Autodesk Inventor part; units mm, degrees
ref_plane "YZ Plane" through (0, 0, 0) normal (1, 0, 0) x (0, 1, 0)
ref_plane "XZ Plane" through (0, 0, 0) normal (0, 1, 0) x (-1, 0, 0)
ref_plane "XY Plane" through (0, 0, 0) normal (0, 0, 1) x (1, 0, 0)
sketch "Skizze_Grudnkörper" plane through (0, 0, 0) normal (0, 0, 1) x (1, 0, 0)
  line L0 (-56, 0) -> (56, 0)
  line L1 (0, -12.6) -> (0, 12.6)
  line L2 (40, -9) -> (-40, -9)
  line L3 (-40, -9) -> (-40, 9)
  line L4 (-40, 9) -> (40, 9)
  line L5 (40, 9) -> (40, -9)
  line L6 (40, -9) -> (-40, 9) construction
  line L7 (-40, -9) -> (40, 9) construction
  point P0 (0, 0)
  dimension "Länge" = 80
  dimension "Breite" = 18
extrude "Grundkörper" add sketch "Skizze_Grudnkörper" along normal blind 10
sketch "Skizze_Senkbohrung" plane through (0, 0, 10) normal (0, 0, 1) x (1, 0, 0)
  line L0 (-56, 0) -> (56, 0)
  line L1 (0, -12.6) -> (0, 12.6)
  line L2 (-40, -9) -> (40, -9)
  line L3 (40, -9) -> (40, 9)
  line L4 (40, 9) -> (-40, 9)
  line L5 (-40, 9) -> (-40, -9)
  point P0 (0, 0)
  point P1 (-35, 0)
  point P2 (35, 0)
  dimension "d4" = 70
hole "Senkbohrung" at (-35, 0, 10) at (35, 0, 10) direction (0, 0, -1) diameter 4.5 end through all counterbore diameter 8 counterbore depth 4.6
sketch "Skizze_Ausnehmung" plane through (0, 0, 0) normal (0, 0, -1) x (-1, 0, 0)
  circle A0 centre (35, 0) radius 2.25
  circle A1 centre (-35, 0) radius 2.25
  line L0 (-40, -9) -> (40, -9)
  line L1 (40, -9) -> (40, 9)
  line L2 (40, 9) -> (-40, 9)
  line L3 (-40, 9) -> (-40, -9)
  line L4 (56, 0) -> (-56, 0)
  line L5 (0, -12.6) -> (0, 12.6)
  line L6 (40, 9) -> (-40, 9)
  line L7 (40, -9) -> (30, -9)
  line L8 (30, -9) -> (30, 9)
  line L9 (30, 9) -> (40, 9)
  line L10 (40, 9) -> (40, -9)
  line L11 (-40, 9) -> (-40, -9)
  line L12 (-40, -9) -> (-30, -9)
  line L13 (-30, -9) -> (-30, 9)
  line L14 (-30, 9) -> (-40, 9)
  line L15 (-40, 9) -> (-40, -9)
  point P0 (0, 0)
  dimension "d12" = 60
extrude "Ausnehmung" cut sketch "Skizze_Ausnehmung" against normal blind 2 contours L4 L1 L0 L8 A0 | A0 L4 L8 L2 L1 | L13 L0 L3 L4 A1 | L4 A1 L3 L2 L13
properties material "Stahl, unlegiert"
Check sheet for the modelled part. Datum: model origin and axes. Units: mm. A direction names the side the tool comes from. Coordinates: 2 decimals unless noted, no trailing zeros. Loops run counter-clockwise (first coordinate to the right, second up) from the corner with the lowest first, then second, coordinate; pieces in that order, holes last.
1) Gauge pin test, flat ends, axial feed: pin 1 (10.5 mm diameter, centred on x = 35, y = 0, fed in from +Z); pin 2 (1.6 mm diameter, centred on y = -0.5, z = 0.5, fed in from -X); pin 3 (7 mm diameter, centred on x = -35, y = 0, fed in from +Z); pin 4 (3 mm diameter, centred on x = -37.5, y = 3.5, fed in from -Z). Record the tip position at first contact, or that the pin passes through.
2) Sectioned sample at C-C (z = 6.75). Record the boundary of the cut face in (x, y).
3) Access from +Z, -Z, +X, -X, +Y, -Y to the whole of each face (thin tool, end or side, straight path). Record for faces 4 (the face through (-33.8, 2.1, 2)), 5 (the face through (37, -2, 5.4)), 6 (the face through (-37.23, 0.29, 3.68)), 7 (the face through (36.2, 2.1, 2)), 8 (the face through (-40, 0, 6)).
4) Release check for a two-part mould opening along Y. For faces 1 (the face through (-30, 0, 1)), 2 (the face through (1, -9, 5)), 3 (the face through (32.77, 0.29, 3.68)) record: released by +Y, released by -Y, zero draft, split by the parting line, or undercut.
5) Sectioned sample at B-B (x = -35). Record the boundary of the cut face in (y, z), and give its area (3 significant figures).
6) Material ranges on probe 1 along X at (y, z) = (0, 6.85); probe 2 along Y at (x, z) = (-35, 2.8); probe 3 along Y at (x, z) = (-35, 8.15), recorded low to high.
7) Sectioned sample at A-A (y = 0). Record the boundary of the cut face in (x, z), and give its area (3 significant figures).
8) Sectioned sample at D-D (z = 1). Record the boundary of the cut face in (x, y).
Check sheet entries:
1. pin 1: stops at z = 10
1. pin 2: stops at x = -30
1. pin 3: stops at z = 5.4
1. pin 4: stops at z = 2
2. outline: (-40, -9) - (40, -9) - (40, 9) - (-40, 9) - close; hole circle Ø8 at (-35, 0); hole circle Ø8 at (35, 0)
3. face 4: -Z, -X, +Y, -Y
3. face 5: +Z
3. face 6: +Z, -Z
3. face 7: -Z, +X, +Y, -Y
3. face 8: +Z, -Z, -X, +Y, -Y
4. face 1: zero draft
4. face 2: released by -Y
4. face 3: undercut
5. outline: (-9, 2) - (-2.25, 2) - (-2.25, 5.4) - (-4, 5.4) - (-4, 10) - (-9, 10) - close; (2.25, 2) - (9, 2) - (9, 10) - (4, 10) - (4, 5.4) - (2.25, 5.4) - close
5. area: 91.9 mm2
6. probe 1: x = -40 to -39, -31 to 31, 39 to 40
6. probe 2: y = -9 to -2.25, 2.25 to 9
6. probe 3: y = -9 to -4, 4 to 9
7. outline: (-40, 2) - (-37.25, 2) - (-37.25, 5.4) - (-39, 5.4) - (-39, 10) - (-40, 10) - close; (-32.75, 2) - (-30, 2) - (-30, 0) - (30, 0) - (30, 2) - (32.75, 2) - (32.75, 5.4) - (31, 5.4) - (31, 10) - (-31, 10) - (-31, 5.4) - (-32.75, 5.4) - close; (37.25, 2) - (40, 2) - (40, 10) - (39, 10) - (39, 5.4) - (37.25, 5.4) - close
7. area: 656 mm2
8. outline: (-30, -9) - (30, -9) - (30, 9) - (-30, 9) - close
